Read the model definition and answer for the solid it produces. Units are mm, in the model's axes. Face numbers are marked on the shaded views. A direction names the side the tool comes from. Give positions to 0.01 mm unless a question says otherwise; leave off trailing zeros. Order: outer loops, then holes, each group sorted by start corner. A loop starts at its lowest first (then second) coordinate and runs counter-clockwise, first axis right, second up. Notation, with made-up numbers: M 24.25,-16 L 76.25,-16 A11 cw 76.25,-4 Z; hole C 64,18.5 d4. An arc over 180 degrees is marked long. Write item = value, one per line. Start each with the question number.
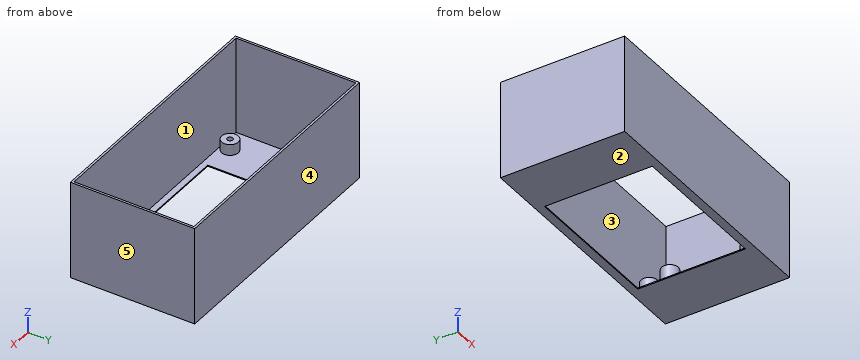
from build123d import *

# Parameters (mm, degrees)
SKETCH_W      = 92
SKETCH_H      = 45
SKETCH_W_2    = 52
SKETCH_H_2    = 39
PAD_DEPTH     = 0.4
SKETCH003_W   = 92
SKETCH003_H   = 45
SKETCH003_W_2 = 90.4
SKETCH003_H_2 = 43.4
PAD001_DEPTH  = 35
SKETCH001_R   = 3
SKETCH001_R_2 = 1
PAD002_DEPTH  = 4
SKETCH004_R   = 3
SKETCH004_R_2 = 1
PAD003_DEPTH  = 15


with BuildPart() as part:
    # Sketch → Pad (new body)
    with BuildSketch(Plane.XY):
        Rectangle(SKETCH_W, SKETCH_H)
        Rectangle(SKETCH_W_2, SKETCH_H_2, mode=Mode.SUBTRACT)
    extrude(amount=-PAD_DEPTH)

    # Sketch003 → Pad001 (join)
    with BuildSketch(Plane.XY):
        Rectangle(SKETCH003_W, SKETCH003_H)
        Rectangle(SKETCH003_W_2, SKETCH003_H_2, mode=Mode.SUBTRACT)
    extrude(amount=PAD001_DEPTH)

    # Sketch001 → Pad002 (join)
    with BuildSketch(Plane.XY):
        with Locations((30.5, 18.25)):
            Circle(SKETCH001_R)
        with Locations((30.5, 18.25)):
            Circle(SKETCH001_R_2, mode=Mode.SUBTRACT)
        with Locations((30.5, -18.25)):
            Circle(SKETCH001_R)
        with Locations((30.5, -18.25)):
            Circle(SKETCH001_R_2, mode=Mode.SUBTRACT)
        with Locations((-36.5, 18.25)):
            Circle(SKETCH001_R)
        with Locations((-36.5, 18.25)):
            Circle(SKETCH001_R_2, mode=Mode.SUBTRACT)
        with Locations((-36.5, -18.25)):
            Circle(SKETCH001_R)
        with Locations((-36.5, -18.25)):
            Circle(SKETCH001_R_2, mode=Mode.SUBTRACT)
    extrude(amount=PAD002_DEPTH)

    # Sketch004 → Pad003 (join)
    with BuildSketch(Plane.XY):
        with Locations((41.348775, 17.78)):
            Circle(SKETCH004_R)
        with Locations((41.348775, 17.78)):
            Circle(SKETCH004_R_2, mode=Mode.SUBTRACT)
        with Locations((41.348775, -17.78)):
            Circle(SKETCH004_R)
        with Locations((41.348775, -17.78)):
            Circle(SKETCH004_R_2, mode=Mode.SUBTRACT)
    extrude(amount=PAD003_DEPTH)


solid = part.part
1) Find section D-D on x = 30.5. Determine the outline of the cut face in (y, z), plus the area to 3 significant figures.
2) Each of these flat-tipped pins is pushed along its axis until it touches: P1, Ø1, axis at x = 41.5, y = 18, coming from the +Z side; P2, Ø1.8, axis at x = 31.5, y = 17.5, coming from the +Z side. Where does it stop, or does it pass through?
3) For the marked faces 1 and 2, determine the directions among +Z, -Z, +X, -X, +Y, -Y from which every point of the face is accessible in a straight line to the end or side of a thin tool.
4) Find section C-C on z = 11. Determine the outline of the cut face in (x, y), plus the area to 3 significant figures.
5) For a pull along Y with two mould halves and no side action, classify the marked faces 3, 4 and 5 as pulls with the +Y half, pulls with the -Y half, needs draft (parallel to the pull), parting line crosses it, or undercut.
6) Find section A-A on y = 13.5. Determine the outline of the cut face in (x, z), plus the area to 3 significant figures.
7) Find the intervals of material crossed by probe 1 along Y at (x, z) = (30.5, 3); probe 2 along Y at (x, z) = (5.5, 8); probe 3 along X at (y, z) = (-1, 18), in increasing order. Write a range as [from, to].
8) Find section B-B on x = -21. Determine the outline of the cut face in (y, z), plus the area to 3 significant figures.
Numbers:
q1.outline = M -22.5,-0.4 L 22.5,-0.4 L 22.5,35 L 21.7,35 L 21.7,0 L 21.25,0 L 21.25,4 L 19.25,4 L 19.25,0 L 17.25,0 L 17.25,4 L 15.25,4 L 15.25,0 L -15.25,0 L -15.25,4 L -17.25,4 L -17.25,0 L -19.25,0 L -19.25,4 L -21.25,4 L -21.25,0 L -21.7,0 L -21.7,35 L -22.5,35 Z
q1.area = 106 mm2
q2.P1 = 0
q2.P2 = 4
q3.face_1 = +Z
q3.face_2 = -Z, +X, -X, +Y, -Y
q4.outline = M -46,-22.5 L 46,-22.5 L 46,22.5 L -46,22.5 Z; C 41.35,-17.78 d6; C 41.35,17.78 d6; hole M -45.2,-21.7 L 45.2,-21.7 L 45.2,21.7 L -45.2,21.7 Z; hole C 41.35,-17.78 d2; hole C 41.35,17.78 d2
q4.area = 267 mm2
q5.face_3 = undercut
q5.face_4 = pulls with the +Y half
q5.face_5 = needs draft
q6.outline = M -46,-0.4 L -26,-0.4 L -26,0 L -45.2,0 L -45.2,35 L -46,35 Z; M 26,-0.4 L 46,-0.4 L 46,35 L 45.2,35 L 45.2,0 L 26,0 Z
q6.area = 72.0 mm2
q7.probe_1 = [-22.5, -21.7], [-21.25, -19.25], [-17.25, -15.25], [15.25, 17.25], [19.25, 21.25], [21.7, 22.5]
q7.probe_2 = [-22.5, -21.7], [21.7, 22.5]
q7.probe_3 = [-46, -45.2], [45.2, 46]
q8.outline = M -22.5,-0.4 L -19.5,-0.4 L -19.5,0 L -21.7,0 L -21.7,35 L -22.5,35 Z; M 19.5,-0.4 L 22.5,-0.4 L 22.5,35 L 21.7,35 L 21.7,0 L 19.5,0 Z
q8.area = 58.4 mm2
